Work out the finished part from the listing and answer in its coordinate system (mm). Give positions to 0.01 mm unless a question says otherwise; leave off trailing zeros. Loops run counter-clockwise (first coordinate to the right, second up) from the corner with the lowest first, then second, coordinate; pieces in that order, holes last. Notation, with made-up numbers: (-37.75, 68) - (-27.75, 68) arc R14 cw to (-27.75, 83) - close; hole circle Ø2 at (-23, 5). An arc over 180 degrees is marked (long way). One line per question, with ' | ' between items. Start each with the question number.
1. Section A-A (z = 0) is taken. Determine the outline of the cut face in (x, y), plus the area to 3 significant figures.
2. Section D-D (x = 5) is taken. Determine the outline of the cut face in (y, z).
3. Section C-C (x = -47) is taken. Determine the outline of the cut face in (y, z), plus the area to 3 significant figures.
4. Find the intervals of material crossed by line 1 (X direction, y = 1, z = 2.1); line 2 (Z direction, x = -18.5, y = -1.5); line 3 (Y direction, x = 35, z = 1.3), in increasing order.
from build123d import *

# Parameters (mm, degrees)
SKETCH1_R           = 2.5
BOSS_EXTRUDE1_DEPTH = 45
SKETCH2_R           = 2.5
SKETCH2_R_2         = 2
CUT_EXTRUDE1_DEPTH  = 8
SKETCH3_R           = 2.5
SKETCH3_R_2         = 2
CUT_EXTRUDE2_DEPTH  = 8
SKETCH4_R           = 2
BOSS_EXTRUDE2_DEPTH = 10
SKETCH5_R           = 2
BOSS_EXTRUDE3_DEPTH = 10


with BuildPart() as part:
    # Sketch1 → Boss-Extrude1 (new body, symmetric)
    with BuildSketch(Plane(origin=(0, 0, 0), x_dir=(0, 0, -1), z_dir=(1, 0, 0))):
        Circle(SKETCH1_R)
    extrude(amount=BOSS_EXTRUDE1_DEPTH, both=True)

    # Sketch2 → Cut-Extrude1 (cut)
    with BuildSketch(Plane(origin=(45, 0, 0), x_dir=(0, 0, -1), z_dir=(1, 0, 0))):
        Circle(SKETCH2_R)
        Circle(SKETCH2_R_2, mode=Mode.SUBTRACT)
    extrude(amount=-CUT_EXTRUDE1_DEPTH, mode=Mode.SUBTRACT)

    # Sketch3 → Cut-Extrude2 (cut)
    with BuildSketch(Plane.ZY.offset(45)):
        Circle(SKETCH3_R)
        Circle(SKETCH3_R_2, mode=Mode.SUBTRACT)
    extrude(amount=-CUT_EXTRUDE2_DEPTH, mode=Mode.SUBTRACT)

    # Sketch4 → Boss-Extrude2 (add)
    with BuildSketch(Plane(origin=(45, 0, 0), x_dir=(0, 0, -1), z_dir=(1, 0, 0))):
        Circle(SKETCH4_R)
    extrude(amount=BOSS_EXTRUDE2_DEPTH)

    # Sketch5 → Boss-Extrude3 (add)
    with BuildSketch(Plane.ZY.offset(45)):
        Circle(SKETCH5_R)
    extrude(amount=BOSS_EXTRUDE3_DEPTH)


solid = part.part
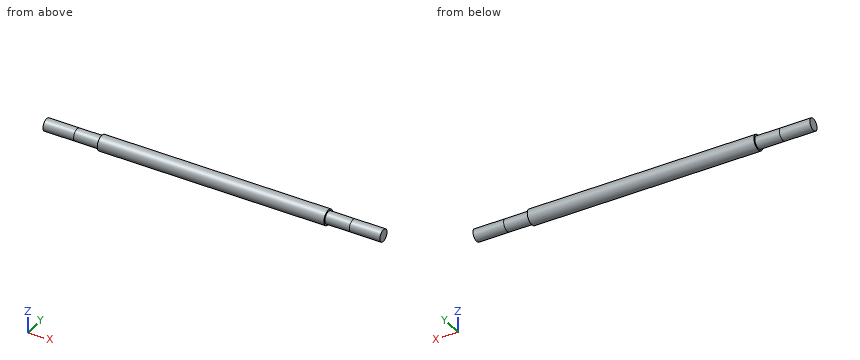
Conclusion:
1) outline: (-55, -2) - (-37, -2) - (-37, -2.5) - (37, -2.5) - (37, -2) - (55, -2) - (55, 2) - (37, 2) - (37, 2.5) - (-37, 2.5) - (-37, 2) - (-55, 2) - close | area: 514 mm²
2) outline: circle Ø5 at (0, 0)
3) outline: circle Ø4 at (0, 0) | area: 12.6 mm²
4) line 1: -37 to 37 | line 2: -2 to 2 | line 3: -2.14 to 2.14
